```python
from build123d import *

# Parameters (mm, degrees)
F1_DEPTH  = 50
F2_R      = 2.5
F3_R      = 9
F4_DEPTH  = 100
F5_R      = 12
F7_DEPTH  = 33.5
F6_R      = 12
F8_DEPTH  = 33.5
F9_R      = 5
F11_DEPTH = 3
F10_R     = 3
F12_DEPTH = 2.5


with BuildPart() as f1:
    # F0 (on Front) → F1 (new body, symmetric)
    with BuildSketch(Plane.XZ):
        with BuildLine():
            Line((27.5, 5.5), (0, 5.5))
            Line((0, 5.5), (0, 0))
            Line((0, 0), (37.3689500386, 0))
            Line((37.3689500386, 0), (38.25, 0.8810499614))
            ThreePointArc((38.25, 0.8810499614), (33.172918626, 3.6252742871), (29.9640842591, 8.4222425415))
            ThreePointArc((29.9640842591, 8.4222425415), (29.4112308016, 6.388417913), (27.5, 5.5))
        make_face()
        with BuildLine():
            ThreePointArc((53.25, 12.5), (39.1800952788, 24.320130898), (29.9640842591, 8.4222425415))
            ThreePointArc((29.9640842591, 8.4222425415), (33.172918626, 3.6252742871), (38.25, 0.8810499614))
            ThreePointArc((38.25, 0.8810499614), (48.5984692283, 3.0131670195), (53.25, 12.5))
        make_face()
    extrude(amount=F1_DEPTH, both=True)

    # F2
    f2_edges = [f1.edges().sort_by_distance(p)[0] for p in [
        (0, 0, 5.5),
    ]]
    fillet(f2_edges, radius=F2_R)

    # F3 (on face) → F4 (cut, through all)
    with BuildSketch(Plane.XZ.offset(50)):
        with Locations((41.25, 12.5)):
            Circle(F3_R)
    extrude(amount=-F4_DEPTH, mode=Mode.SUBTRACT)

    # F5 (on face) → F7 (cut)
    with BuildSketch(Plane.XZ.offset(50)):
        with Locations((41.25, 12.5)):
            Circle(F5_R)
    extrude(amount=-F7_DEPTH, mode=Mode.SUBTRACT)

    # F6 (on face) → F8 (cut)
    with BuildSketch(Plane(origin=(0, 50, 0), x_dir=(-1, 0, 0), z_dir=(0, 1, 0))):
        with Locations((-41.25, 12.5)):
            Circle(F6_R)
    extrude(amount=-F8_DEPTH, mode=Mode.SUBTRACT)

    # F9 (on face) → F11 (cut)
    with BuildSketch(Plane.XY.offset(5.5)):
        with Locations((15, 0)):
            Circle(F9_R)
        with Locations((15, 37)):
            Circle(F9_R)
        with Locations((15, -37)):
            Circle(F9_R)
    extrude(amount=-F11_DEPTH, mode=Mode.SUBTRACT)

    # F10 (on face) → F12 (cut, through all)
    with BuildSketch(Plane(origin=(0, 0, 0), x_dir=(1, 0, 0), z_dir=(0, 0, -1))):
        with Locations((15, -37)):
            Circle(F10_R)
        with Locations((15, 0)):
            Circle(F10_R)
        with Locations((15, 37)):
            Circle(F10_R)
    extrude(amount=-F12_DEPTH, mode=Mode.SUBTRACT)


solid = f1.part
```
The model under review builds one solid part; all positions refer to its coordinate system, in mm. A direction names the side the tool comes from. Coordinates: 2 decimals unless noted, no trailing zeros. Write each loop counter-clockwise with the first axis right and the second up, starting at its lowest first coordinate (ties: lowest second). Pieces come first, ordered by that corner, then holes. Notation, with made-up numbers: (-12, -17.75) - (43, -17.75) arc R24 ccw to (43, 19.25) - close; hole circle Ø2 at (-19.75, 2.25). An arc over 180 degrees is marked (long way). Answer in a Markdown table with one row per item. Add a question column.
Q1. Consider section D-D on y = 20.5. Give the boundary of the cut face in (x, z), then the cut area to 3 significant figures.
Q2. Draft analysis for pull direction Z (two halves, no side actions). For faces 4 (the face through (18, -1, 0)), 5 (the face through (34.11, -0.23, 7.02)), 6 (the face through (19, -50, 2)), 7 (the face through (14.9, -3.3, 2.5)), state which applies: +Z half, -Z half, draft (parallel to the pull), parting line (faces both ways), or undercut.
Q3. For faces 1 (the face through (33.2, 33.5, 3.6)), 2 (the face through (14.9, 33.7, 2.5)), 3 (the face through (46, -16.5, 21)), list the 3-axis set-ups (+Z, -Z, +X, -X, +Y, -Y) from which the entire face can be reached by the end or side of a thin tool; tool diameter is ignored.
Q4. Consider section C-C on x = 15. Give the boundary of the cut face in (y, z).
Q5. Consider section A-A on x = 41.25. Give the boundary of the cut face in (y, z).
Q6. To check wall thickness, follow line 1 along Z through (x, y) = (41.25, 8.5); line 2 along Y through (x, z) = (15, 4.6); line 3 along Z through (x, y) = (13.5, 43.5). State the ranges of each line that lie inside material, in increasing order. Write a range as from..to.
Q7. Consider section B-B on y = 37. Give the boundary of the cut face in (x, z).
Q8. Clearance check with flat-ended pins moving along their axes: pin 1 (9.5 mm diameter, centred on x = 15, y = 0, fed in from +Z); pin 2 (1.5 mm diameter, centred on x = 42, y = -2.5, fed in from +Z); pin 3 (1.5 mm diameter, centred on y = 30, z = 7, fed in from +X); pin 4 (3 mm diameter, centred on x = 6.5, y = 4, fed in from +Z). State where each tip first meets the part, or that it passes through.
Answers below:
| question | item | result |
|---|---|---|
| 1 | outline | (0, 0) - (37.37, 0) - (38.25, 0.88) arc R12 cw to (29.96, 8.42) arc R2.5 cw to (27.5, 5.5) - (2.5, 5.5) arc R2.5 ccw to (0, 3) - close |
| 1 | area | 192 mm² |
| 2 | face 4 | -Z half |
| 2 | face 5 | undercut |
| 2 | face 6 | draft |
| 2 | face 7 | +Z half |
| 3 | face 1 | +Z, +X, +Y |
| 3 | face 2 | +Z |
| 3 | face 3 | +Z, +X, -Y |
| 4 | outline | (-50, 0) - (-40, 0) - (-40, 2.5) - (-42, 2.5) - (-42, 5.5) - (-50, 5.5) - close; (-34, 0) - (-3, 0) - (-3, 2.5) - (-5, 2.5) - (-5, 5.5) - (-32, 5.5) - (-32, 2.5) - (-34, 2.5) - close; (3, 0) - (34, 0) - (34, 2.5) - (32, 2.5) - (32, 5.5) - (5, 5.5) - (5, 2.5) - (3, 2.5) - close; (40, 0) - (50, 0) - (50, 5.5) - (42, 5.5) - (42, 2.5) - (40, 2.5) - close |
| 5 | outline | (-16.5, 0.5) - (16.5, 0.5) - (16.5, 3.5) - (-16.5, 3.5) - close; (-16.5, 21.5) - (16.5, 21.5) - (16.5, 24.5) - (-16.5, 24.5) - close |
| 6 | line 1 | 0.5..3.5, 21.5..24.5 |
| 6 | line 2 | -50..-42, -32..-5, 5..32, 42..50 |
| 6 | line 3 | 0..5.5 |
| 7 | outline | (0, 0) - (12, 0) - (12, 2.5) - (10, 2.5) - (10, 5.5) - (2.5, 5.5) arc R2.5 ccw to (0, 3) - close; (18, 0) - (37.37, 0) - (38.25, 0.88) arc R12 cw to (29.96, 8.42) arc R2.5 cw to (27.5, 5.5) - (20, 5.5) - (20, 2.5) - (18, 2.5) - close |
| 8 | pin 1 | z = 2.5 |
| 8 | pin 2 | z = 24.5 |
| 8 | pin 3 | x = 31.01 |
| 8 | pin 4 | z = 5.5 |
